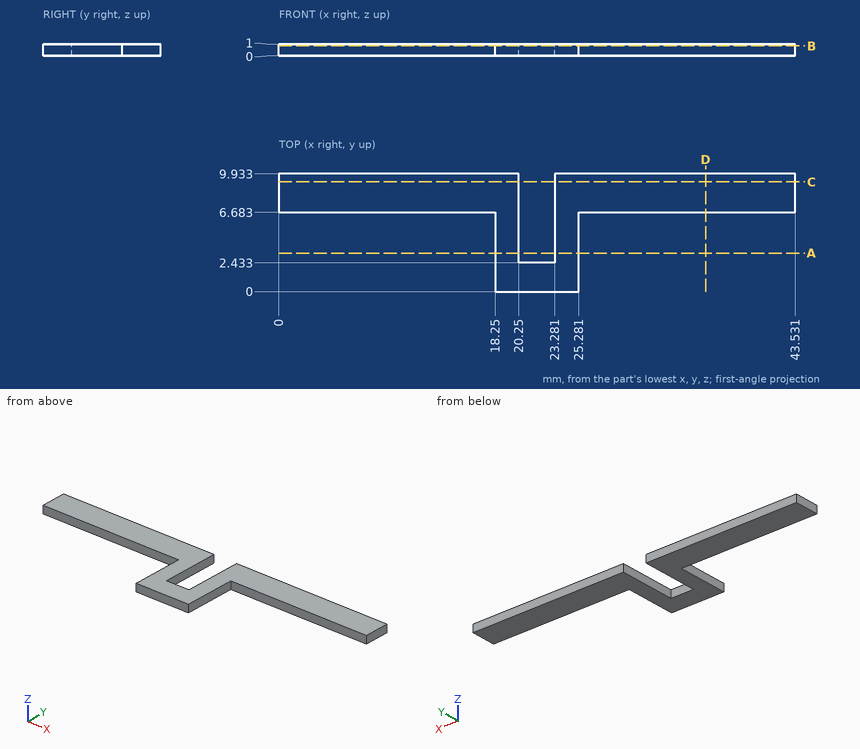
Geometry: see drawing. Coordinates: mm, zero at the bounding-box minimum. Give positions to 0.01 mm unless a question says otherwise; leave off trailing zeros. Order: outer loops, then holes, each group sorted by start corner. A loop starts at its lowest first (then second) coordinate and runs counter-clockwise, first axis right, second up. Notation, with made-up numbers: (2, -23) -> (52, -23) arc R12 cw to (52, -1) -> close; hole circle Ø2 at (25.5, 56.25). An arc over 180 degrees is marked (long way). Write each question's results on one line, items separated by ' | '.
1) Cut plane C-C (y = 9.25). Output: boundary loops of the cut face in (x, z), and give its area (3 significant figures).
Geometry says:
outline: (0, 0) -> (20.25, 0) -> (20.25, 1) -> (0, 1) -> close; (23.28, 0) -> (43.53, 0) -> (43.53, 1) -> (23.28, 1) -> close | area: 40.5 mm²
2) Cut plane D-D (x = 36). Output: boundary loops of the cut face in (y, z).
Geometry says:
outline: (6.68, 0) -> (9.93, 0) -> (9.93, 1) -> (6.68, 1) -> close
3) Line query: line 1 along X through (y, z) = (4.5, 0.3); line 2 along X through (y, z) = (7, 0.5); line 3 along Y through (x, z) = (29.5, 0.35). Output: solid intervals per line, ascending.
Geometry says:
line 1: x = 18.25 to 20.25, 23.28 to 25.28 | line 2: x = 0 to 20.25, 23.28 to 43.53 | line 3: y = 6.68 to 9.93
4) Cut plane A-A (y = 3.25). Output: boundary loops of the cut face in (x, z).
Geometry says:
outline: (18.25, 0) -> (20.25, 0) -> (20.25, 1) -> (18.25, 1) -> close; (23.28, 0) -> (25.28, 0) -> (25.28, 1) -> (23.28, 1) -> close
5) First-contact query: pin 1 Ø0.5 at (x, z) = (36.5, 0.5) entering from -Y. Flat tip, straight axial feed; report the tip coordinate or a pass-through.
Geometry says:
pin 1: stops at y = 6.68
6) Cut plane B-B (z = 0.85). Output: boundary loops of the cut face in (x, y), and give its area (3 significant figures).
Geometry says:
outline: (0, 6.68) -> (18.25, 6.68) -> (18.25, 0) -> (25.28, 0) -> (25.28, 6.68) -> (43.53, 6.68) -> (43.53, 9.93) -> (23.28, 9.93) -> (23.28, 2.43) -> (20.25, 2.43) -> (20.25, 9.93) -> (0, 9.93) -> close | area: 166 mm²
